from build123d import *

# Parameters (mm, degrees)
EXTRUDE_1_DEPTH     = 3
SKETCH_2_W          = 37
SKETCH_2_H          = 3
EXTRUDE_2_DEPTH     = 6.5
SKETCH_3_W          = 20
SKETCH_3_H          = 4
CUT_EXTRUDE_1_DEPTH = 5
FILLET_2_R          = 3
EXTRUDE_START       = -3
EXTRUDE_4_DEPTH     = 3


with BuildPart() as part:
    # Sketch 1 → Extrude 1 (new body)
    with BuildSketch(Plane.XY):
        with BuildLine():
            Line((18.5, 23.5), (-18.5, 23.5))
            ThreePointArc((-18.5, 23.5), (-22.035533906, 22.035533906), (-23.5, 18.5))
            Line((-23.5, 18.5), (-23.5, -18.5))
            ThreePointArc((-23.5, -18.5), (-22.035533906, -22.035533906), (-18.5, -23.5))
            Line((-18.5, -23.5), (18.5, -23.5))
            ThreePointArc((18.5, -23.5), (22.035533906, -22.035533906), (23.5, -18.5))
            Line((23.5, -18.5), (23.5, 18.5))
            ThreePointArc((23.5, 18.5), (22.035533906, 22.035533906), (18.5, 23.5))
        make_face()
        with BuildLine():
            Line((-12.196084122, 8.732441359), (-19.231821381, 15.768178619))
            ThreePointArc((-19.231821381, 15.768178619), (-19.231821381, 19.231821381), (-15.768178619, 19.231821381))
            Line((-15.768178619, 19.231821381), (-8.732441359, 12.196084122))
            ThreePointArc((-8.732441359, 12.196084122), (0, 15), (8.732441359, 12.196084122))
            Line((8.732441359, 12.196084122), (15.768178619, 19.231821381))
            ThreePointArc((15.768178619, 19.231821381), (19.231821381, 19.231821381), (19.231821381, 15.768178619))
            Line((19.231821381, 15.768178619), (12.196084122, 8.732441359))
            ThreePointArc((12.196084122, 8.732441359), (15, 0), (12.196084122, -8.732441359))
            Line((12.196084122, -8.732441359), (19.231821381, -15.768178619))
            ThreePointArc((19.231821381, -15.768178619), (19.231821381, -19.231821381), (15.768178619, -19.231821381))
            Line((15.768178619, -19.231821381), (8.732441359, -12.196084122))
            ThreePointArc((8.732441359, -12.196084122), (0, -15), (-8.732441359, -12.196084122))
            Line((-8.732441359, -12.196084122), (-15.768178619, -19.231821381))
            ThreePointArc((-15.768178619, -19.231821381), (-19.231821381, -19.231821381), (-19.231821381, -15.768178619))
            Line((-19.231821381, -15.768178619), (-12.196084122, -8.732441359))
            ThreePointArc((-12.196084122, -8.732441359), (-15, 0), (-12.196084122, 8.732441359))
        make_face(mode=Mode.SUBTRACT)
    extrude(amount=EXTRUDE_1_DEPTH)

    # Sketch 2 → Extrude 2 (add)
    with BuildSketch(Plane(origin=(0, 23.5, 0), x_dir=(1, 0, 0), z_dir=(0, 1, 0))):
        with Locations((0, -1.5)):
            Rectangle(SKETCH_2_W, SKETCH_2_H)
    extrude(amount=EXTRUDE_2_DEPTH)

    # Sketch 3 → Cut-Extrude 1 (cut)
    with BuildSketch(Plane.XY.offset(3)):
        with Locations((0, 25.5)):
            Rectangle(SKETCH_3_W, SKETCH_3_H)
    extrude(amount=-CUT_EXTRUDE_1_DEPTH, mode=Mode.SUBTRACT)

    # Fillet 2
    fillet_2_edges = [part.edges().sort_by_distance(p)[0] for p in [
        (18.5, 23.5, 1.5),
        (-18.5, 23.5, 1.5),
        (-18.5, 30, 1.5),
        (18.5, 30, 1.5),
    ]]
    fillet(fillet_2_edges, radius=FILLET_2_R)

    # Sketch 5 → Extrude 4 (add)
    with BuildSketch(Plane.XY.offset(3).offset(EXTRUDE_START)):
        with BuildLine():
            ThreePointArc((-15.768178619, 19.231821381), (-19.231821381, 19.231821381), (-19.231821381, 15.768178619))
            Line((-19.231821381, 15.768178619), (-12.196084122, 8.732441359))
            ThreePointArc((-12.196084122, 8.732441359), (-11.911158294, 9.11725332), (-11.614095631, 9.492775288))
            Line((-11.614095631, 9.492775288), (-18.560660172, 16.439339828))
            ThreePointArc((-18.560660172, 16.439339828), (-18.560660172, 18.560660172), (-16.439339828, 18.560660172))
            Line((-16.439339828, 18.560660172), (-9.492775288, 11.614095631))
            ThreePointArc((-9.492775288, 11.614095631), (-9.11725332, 11.911158294), (-8.732441359, 12.196084122))
            Line((-8.732441359, 12.196084122), (-15.768178619, 19.231821381))
        make_face()
        with BuildLine():
            Line((15.768178619, 19.231821381), (8.732441359, 12.196084122))
            ThreePointArc((8.732441359, 12.196084122), (9.11725332, 11.911158294), (9.492775288, 11.614095631))
            Line((9.492775288, 11.614095631), (16.439339828, 18.560660172))
            ThreePointArc((16.439339828, 18.560660172), (18.074025149, 18.885819299), (19, 17.5))
            ThreePointArc((19, 17.5), (18.885819299, 16.925974851), (18.560660172, 16.439339828))
            Line((18.560660172, 16.439339828), (11.614095631, 9.492775288))
            ThreePointArc((11.614095631, 9.492775288), (11.911158294, 9.11725332), (12.196084122, 8.732441359))
            Line((12.196084122, 8.732441359), (19.231821381, 15.768178619))
            ThreePointArc((19.231821381, 15.768178619), (19.231821381, 19.231821381), (15.768178619, 19.231821381))
        make_face()
        with BuildLine():
            ThreePointArc((-11.614095631, -9.492775288), (-11.911158294, -9.11725332), (-12.196084122, -8.732441359))
            Line((-12.196084122, -8.732441359), (-19.231821381, -15.768178619))
            ThreePointArc((-19.231821381, -15.768178619), (-19.231821381, -19.231821381), (-15.768178619, -19.231821381))
            Line((-15.768178619, -19.231821381), (-8.732441359, -12.196084122))
            ThreePointArc((-8.732441359, -12.196084122), (-9.11725332, -11.911158294), (-9.492775288, -11.614095631))
            Line((-9.492775288, -11.614095631), (-16.439339828, -18.560660172))
            ThreePointArc((-16.439339828, -18.560660172), (-18.560660172, -18.560660172), (-18.560660172, -16.439339828))
            Line((-18.560660172, -16.439339828), (-11.614095631, -9.492775288))
        make_face()
        with BuildLine():
            ThreePointArc((9.492775288, -11.614095631), (9.11725332, -11.911158294), (8.732441359, -12.196084122))
            Line((8.732441359, -12.196084122), (15.768178619, -19.231821381))
            ThreePointArc((15.768178619, -19.231821381), (19.231821381, -19.231821381), (19.231821381, -15.768178619))
            Line((19.231821381, -15.768178619), (12.196084122, -8.732441359))
            ThreePointArc((12.196084122, -8.732441359), (11.911158294, -9.11725332), (11.614095631, -9.492775288))
            Line((11.614095631, -9.492775288), (18.560660172, -16.439339828))
            ThreePointArc((18.560660172, -16.439339828), (18.885819299, -16.925974851), (19, -17.5))
            ThreePointArc((19, -17.5), (18.074025149, -18.885819299), (16.439339828, -18.560660172))
            Line((16.439339828, -18.560660172), (9.492775288, -11.614095631))
        make_face()
    extrude(amount=EXTRUDE_4_DEPTH)


solid = part.part
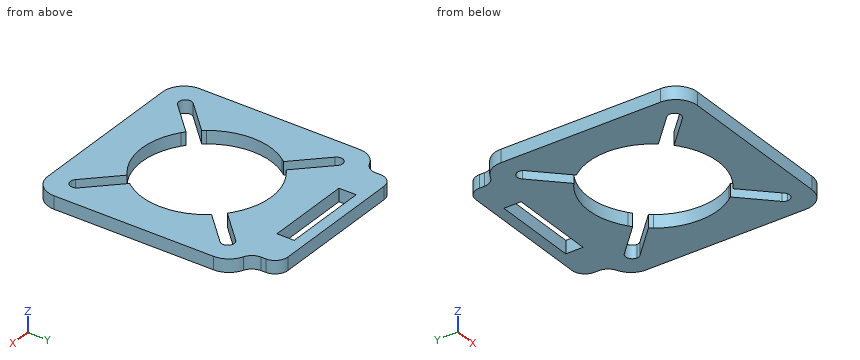
For this review, take the finished solid that the model builds, in its own axes (mm). Coordinates: 2 decimals unless noted, no trailing zeros. Loops run counter-clockwise (first coordinate to the right, second up) from the corner with the lowest first, then second, coordinate; pieces in that order, holes last. Notation, with made-up numbers: (66.25, -37) -> (118.25, -37) arc R19 cw to (118.25, -12) -> close; hole circle Ø8 at (-20.75, -32). An arc over 180 degrees is marked (long way). Write each question's results on one line, items separated by ' | '.
Q1. Add section A-A, the plane x = -17.5. State the section outline as (y, z) points.
Taken from the geometry:
outline: (-23.5, 0) -> (-19, 0) -> (-19, 3) -> (-23.5, 3) -> close; (-15.38, 0) -> (15.38, 0) -> (15.38, 3) -> (-15.38, 3) -> close; (19, 0) -> (29.24, 0) -> (29.24, 3) -> (19, 3) -> close
Q2. To check wall thickness, follow line 1 along Y through (x, z) = (0.5, 2.95); line 2 along X through (y, z) = (0, 2); line 3 along X through (y, z) = (26, 0.3). State the ranges of each line that lie inside material, in increasing order. Write a range as [from, to].
Taken from the geometry:
line 1: [-23.5, -14.99], [14.99, 23.5], [27.5, 30] | line 2: [-23.5, -15], [15, 23.5] | line 3: [-18.5, -10], [10, 18.5]
Q3. For pin 1 Ø0.9 at (y, z) = (26, 2) entering from +X; pin 2 Ø0.5 at (y, z) = (26.5, 1.5) entering from -X, all flat-tipped, find the tip position at first contact; note any pin that passes through.
Taken from the geometry:
pin 1: x = 18.52 | pin 2: x = -18.5
Q4. Add section B-B, the plane y = -7.5. State the section outline as (x, z) points.
Taken from the geometry:
outline: (-23.5, 0) -> (-12.99, 0) -> (-12.99, 3) -> (-23.5, 3) -> close; (12.99, 0) -> (23.5, 0) -> (23.5, 3) -> (12.99, 3) -> close
Q5. Add section C-C, the plane y = -13.5. State the section outline as (x, z) points.
Taken from the geometry:
outline: (-23.5, 0) -> (-15.62, 0) -> (-15.62, 3) -> (-23.5, 3) -> close; (-11.38, 0) -> (-6.54, 0) -> (-6.54, 3) -> (-11.38, 3) -> close; (6.54, 0) -> (11.38, 0) -> (11.38, 3) -> (6.54, 3) -> close; (15.62, 0) -> (23.5, 0) -> (23.5, 3) -> (15.62, 3) -> close
Q6. Add section D-D, the plane z = 0.9. Count the separate pieces of the cut face and the enclosed holes in it, then the cut area to 3 significant figures.
Taken from the geometry:
separate pieces: 1 | enclosed holes: 2 | area: 1,510 mm²
